Verification items for the finished model (mm, model axes). Face numbers are marked on the shaded views. A direction names the side the tool comes from. Round coordinates to 2 decimals unless told otherwise and drop trailing zeros. Order: outer loops, then holes, each group sorted by start corner. A loop starts at its lowest first (then second) coordinate and runs counter-clockwise, first axis right, second up. Notation, with made-up numbers: M 13.25,26 L 40.25,26 A20 cw 40.25,63 Z; hole C 75,22.5 d8. An arc over 180 degrees is marked long. Use one line per item in the form item = value. Start each with the question number.
Item 1: Go/stop test with a flat-tipped pin: pin 1 Ø1.8 at (x, y) = (0, 37) entering from -Z. Record where the tip stops, or that it passes through.
Item 2: Cross-section at C-C on x = 0. Count the separate pieces of the cut face and the enclosed holes in it, then the cut area to 3 significant figures.
Item 3: Cross-section at A-A on x = 4.75. Enter the section's corners in (y, z).
Item 4: Cross-section at B-B on y = 55. Enter the section's corners in (x, z), then the cut area to 3 significant figures.
Item 5: Cross-section at D-D on z = 0. Enter the section's corners in (x, y), then the cut area to 3 significant figures.
Item 6: Thickness scan on probe 1 along Y at (x, z) = (0, -6.95); probe 2 along X at (y, z) = (63.5, -4.25). Record the ranges inside material, lowest first. Write a range as [from, to].
Item 7: Release check for a two-part mould opening along Z. For the marked faces 3, 4 and 5 record: +Z half, -Z half, draft (parallel to the pull), parting line (faces both ways), or undercut.
Item 8: Tool access check on the marked faces 1 and 2. Record the directions out of +Z, -Z, +X, -X, +Y, -Y that give a thin tool (end or side, any length) a straight path to the whole face; none if there is none.
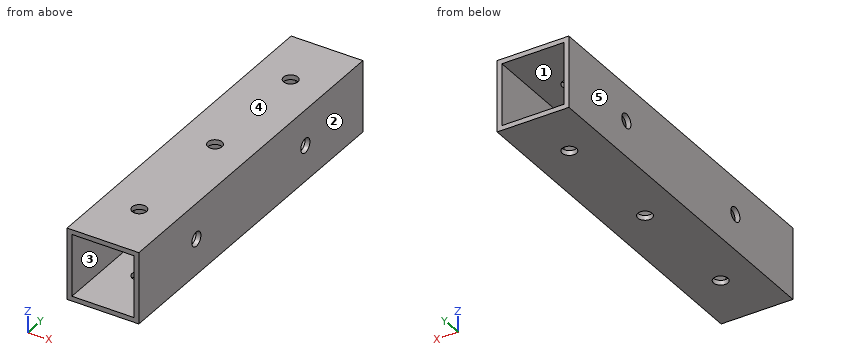
from build123d import *

# Parameters (mm, degrees)
SKETCH_1_W          = 15
SKETCH_1_H          = 15
SKETCH_1_W_2        = 13
SKETCH_1_H_2        = 13
EXTRUDE_1_DEPTH     = 74
SKETCH_2_R          = 1.5
CUT_EXTRUDE_1_DEPTH = 76.876544465
SKETCH_3_R          = 1.5
CUT_EXTRUDE_2_DEPTH = 76.876544465


with BuildPart() as part:
    # 草图1 → 凸台-拉伸1 (new body)
    with BuildSketch(Plane(origin=(0, 0, 0), x_dir=(1, 0, 0), z_dir=(0, 1, 0))):
        Rectangle(SKETCH_1_W, SKETCH_1_H)
        Rectangle(SKETCH_1_W_2, SKETCH_1_H_2, mode=Mode.SUBTRACT)
    extrude(amount=EXTRUDE_1_DEPTH)

    # 草图2 → 切除-拉伸1 (cut, through all)
    with BuildSketch(Plane.XY.offset(7.5)):
        with Locations((0, 62)):
            Circle(SKETCH_2_R)
        with Locations((0, 37)):
            Circle(SKETCH_2_R)
        with Locations((0, 12)):
            Circle(SKETCH_2_R)
    extrude(amount=-CUT_EXTRUDE_1_DEPTH, mode=Mode.SUBTRACT)

    # 草图3 → 切除-拉伸2 (cut, through all)
    with BuildSketch(Plane(origin=(7.5, 0, 0), x_dir=(0, 0, -1), z_dir=(1, 0, 0))):
        with Locations((0, 55)):
            Circle(SKETCH_3_R)
        with Locations((0, 19)):
            Circle(SKETCH_3_R)
    extrude(amount=-CUT_EXTRUDE_2_DEPTH, mode=Mode.SUBTRACT)


solid = part.part
Output values:
q1.pin_1 = through
q2.separate_pieces = 8
q2.enclosed_holes = 0
q2.area = 130 mm2
q3.outline = M 0,-7.5 L 74,-7.5 L 74,-6.5 L 0,-6.5 Z; M 0,6.5 L 74,6.5 L 74,7.5 L 0,7.5 Z
q4.outline = M -7.5,-7.5 L 7.5,-7.5 L 7.5,-1.5 L 6.5,-1.5 L 6.5,-6.5 L -6.5,-6.5 L -6.5,-1.5 L -7.5,-1.5 Z; M -7.5,1.5 L -6.5,1.5 L -6.5,6.5 L 6.5,6.5 L 6.5,1.5 L 7.5,1.5 L 7.5,7.5 L -7.5,7.5 Z
q4.area = 50.0 mm2
q5.outline = M -7.5,0 L -6.5,0 L -6.5,17.5 L -7.5,17.5 Z; M -7.5,20.5 L -6.5,20.5 L -6.5,53.5 L -7.5,53.5 Z; M -7.5,56.5 L -6.5,56.5 L -6.5,74 L -7.5,74 Z; M 6.5,0 L 7.5,0 L 7.5,17.5 L 6.5,17.5 Z; M 6.5,20.5 L 7.5,20.5 L 7.5,53.5 L 6.5,53.5 Z; M 6.5,56.5 L 7.5,56.5 L 7.5,74 L 6.5,74 Z
q5.area = 136 mm2
q6.probe_1 = [0, 10.5], [13.5, 35.5], [38.5, 60.5], [63.5, 74]
q6.probe_2 = [-7.5, -6.5], [6.5, 7.5]
q7.face_3 = undercut
q7.face_4 = +Z half
q7.face_5 = draft
q8.face_1 = +Y, -Y
q8.face_2 = +Z, -Z, +X, +Y, -Y
